```python
from build123d import *

# Parameters (mm, degrees)
SKETCH2_W                   = 42
SKETCH2_H                   = 42
MAIN_BOSS_DEPTH             = 33.75
SKETCH4_W                   = 8.7
SKETCH4_H                   = 17
SIDE_EXTRUDE_DEPTH          = 10
SKETCH5_R                   = 16.5
BIG_CIRCLE_CUT_DEPTH        = 0.5
SKETCH6_R                   = 11
MEDIUM_CIRCLE_EXTRUDE_DEPTH = 2.5
SKETCH7_R                   = 3.5
SMALL_CIRCLE_CUT_DEPTH      = 5
SKETCH8_R                   = 2.25
CIRCULAR_TALL_EXTRUDE_DEPTH = 23
SIDE_EDGE_CUT_DEPTH         = 50.62008162
MIRROR2_DEPTH               = 33.75
SKETCH10_R                  = 1.5
F_4_HOLES_DEPTH             = 5
MIRROR4_COPY_1_SKETCH_R     = 1.5
MIRROR4_COPY_1_DEPTH        = 5
MIRROR6_COPY_1_SKETCH_R     = 1.5
MIRROR6_COPY_1_DEPTH        = 5
MIRROR6_COPY_2_SKETCH_R     = 1.5
MIRROR6_COPY_2_DEPTH        = 5
MIRROR6_COPY_3_SKETCH_R     = 1.5
MIRROR6_COPY_3_DEPTH        = 5
SKETCH12_OUTSIDE_W          = 69.698
SKETCH12_OUTSIDE_H          = 60.998
CUT_AROUND_BODY_DEPTH       = 21


# Read off the part's stored shape, not the designer's step: Mirror2
with BuildPart() as part:
    # Sketch2 → Main Boss (new body)
    with BuildSketch(Plane(origin=(0, 0, 0), x_dir=(1, 0, 0), z_dir=(0, 1, 0))):
        Rectangle(SKETCH2_W, SKETCH2_H)
    extrude(amount=MAIN_BOSS_DEPTH)

    # Sketch4 → side extrude (add)
    with BuildSketch(Plane(origin=(0, 0, 0), x_dir=(1, 0, 0), z_dir=(0, 1, 0))):
        with Locations((25.35, 0)):
            Rectangle(SKETCH4_W, SKETCH4_H)
    extrude(amount=SIDE_EXTRUDE_DEPTH)

    # Sketch5 → Big circle cut (cut)
    with BuildSketch(Plane(origin=(0, 33.75, 0), x_dir=(1, 0, 0), z_dir=(0, 1, 0))):
        with Locations(Location((0, 0, 0), (0, 0, 270))):
            Circle(SKETCH5_R)
    extrude(amount=-BIG_CIRCLE_CUT_DEPTH, mode=Mode.SUBTRACT)

    # Sketch6 → medium circle extrude (add)
    with BuildSketch(Plane(origin=(0, 33.25, 0), x_dir=(1, 0, 0), z_dir=(0, 1, 0))):
        with Locations(Location((0, 0, 0), (0, 0, 270))):
            Circle(SKETCH6_R)
    extrude(amount=MEDIUM_CIRCLE_EXTRUDE_DEPTH)

    # Sketch7 → small circle cut (cut)
    with BuildSketch(Plane(origin=(0, 35.75, 0), x_dir=(1, 0, 0), z_dir=(0, 1, 0))):
        with Locations(Location((0, 0, 0), (0, 0, 270))):
            Circle(SKETCH7_R)
    extrude(amount=-SMALL_CIRCLE_CUT_DEPTH, mode=Mode.SUBTRACT)

    # Sketch8 → circular tall extrude (add)
    with BuildSketch(Plane(origin=(0, 30.75, 0), x_dir=(1, 0, 0), z_dir=(0, 1, 0))):
        with Locations(Location((0, 0, 0), (0, 0, 270))):
            Circle(SKETCH8_R)
    extrude(amount=CIRCULAR_TALL_EXTRUDE_DEPTH)

    # Sketch9 → side edge cut (cut, symmetric)
    with BuildSketch(Plane(origin=(0, 33.75, 0), x_dir=(1, 0, 0), z_dir=(0, 1, 0))):
        Polygon((79.674907888, 117.679754574), (-17.004846686, 21), (-21, 17.004846686), (-117.679754574, -79.674907888), (-311.039263723, 113.684601261), (-113.684601261, 311.039263723), align=None)
    side_edge_cut = extrude(amount=SIDE_EDGE_CUT_DEPTH, both=True, mode=Mode.SUBTRACT)

    # Mirror1: side edge cut across plane
    add(side_edge_cut.mirror(Plane.XY), mode=Mode.SUBTRACT)

    # Mirror2 outline → Mirror2 (cut)
    with BuildSketch(Plane(origin=(0, 0, 0), x_dir=(1, 0, 0), z_dir=(0, 1, 0))):
        Polygon((21, -21), (21, -17.004846686), (17.004846686, -21), align=None)
        Polygon((17.004846686, 21), (21, 17.004846686), (21, 21), align=None)
    extrude(amount=MIRROR2_DEPTH, mode=Mode.SUBTRACT)

    # Sketch10 → 4 holes (cut)
    with BuildSketch(Plane(origin=(0, 33.75, 0), x_dir=(1, 0, 0), z_dir=(0, 1, 0))):
        with Locations(Location((-15.5, 15.5, 0), (0, 0, 270))):
            Circle(SKETCH10_R)
    f_4_holes = extrude(amount=-F_4_HOLES_DEPTH, mode=Mode.SUBTRACT)

    # Mirror3: 4 holes across plane
    add(f_4_holes.mirror(Plane.XY), mode=Mode.SUBTRACT)

    # Mirror4: 4 holes across plane
    add(f_4_holes.mirror(Plane(origin=(0, 0, 0), x_dir=(0, 0, 1), z_dir=(1, 0, 0))), mode=Mode.SUBTRACT)

    # Mirror4 copy 1 sketch → Mirror4 copy 1 (cut)
    with BuildSketch(Plane(origin=(0, 33.75, 0), x_dir=(-1, 0, 0), z_dir=(0, 1, 0))):
        with Locations(Location((-15.5, 15.5, 0), (0, 0, 270))):
            Circle(MIRROR4_COPY_1_SKETCH_R)
    extrude(amount=-MIRROR4_COPY_1_DEPTH, mode=Mode.SUBTRACT)

    # Mirror6: 4 holes across plane
    add(f_4_holes.mirror(Plane.ZX.offset(16.875)), mode=Mode.SUBTRACT)

    # Mirror6 copy 1 sketch → Mirror6 copy 1 (cut)
    with BuildSketch(Plane.XZ):
        with Locations(Location((-15.5, 15.5, 0), (0, 0, 270))):
            Circle(MIRROR6_COPY_1_SKETCH_R)
    extrude(amount=-MIRROR6_COPY_1_DEPTH, mode=Mode.SUBTRACT)

    # Mirror6 copy 2 sketch → Mirror6 copy 2 (cut)
    with BuildSketch(Plane(origin=(0, 0, 0), x_dir=(-1, 0, 0), z_dir=(0, -1, 0))):
        with Locations(Location((-15.5, 15.5, 0), (0, 0, 270))):
            Circle(MIRROR6_COPY_2_SKETCH_R)
    extrude(amount=-MIRROR6_COPY_2_DEPTH, mode=Mode.SUBTRACT)

    # Mirror6 copy 3 sketch → Mirror6 copy 3 (cut)
    with BuildSketch(Plane(origin=(0, 0, 0), x_dir=(-1, 0, 0), z_dir=(0, -1, 0))):
        with Locations((-15.5, -15.5)):
            Circle(MIRROR6_COPY_3_SKETCH_R)
    extrude(amount=-MIRROR6_COPY_3_DEPTH, mode=Mode.SUBTRACT)

    # Sketch12 outside → cut around body (cut)
    with BuildSketch(Plane(origin=(0, 7, 0), x_dir=(1, 0, 0), z_dir=(0, 1, 0))):
        with Locations((4.35, 0)):
            Rectangle(SKETCH12_OUTSIDE_W, SKETCH12_OUTSIDE_H)
        with BuildLine():
            Line((-15.5, -19.5), (15.5, -19.5))
            ThreePointArc((15.5, -19.5), (18.328427125, -18.328427125), (19.5, -15.5))
            Line((19.5, -15.5), (19.5, 15.5))
            ThreePointArc((19.5, 15.5), (18.328427125, 18.328427125), (15.5, 19.5))
            Line((15.5, 19.5), (-15.5, 19.5))
            ThreePointArc((-15.5, 19.5), (-18.328427125, 18.328427125), (-19.5, 15.5))
            Line((-19.5, 15.5), (-19.5, -15.5))
            ThreePointArc((-19.5, -15.5), (-18.328427125, -18.328427125), (-15.5, -19.5))
        make_face(mode=Mode.SUBTRACT)
    extrude(amount=CUT_AROUND_BODY_DEPTH, mode=Mode.SUBTRACT)


solid = part.part
```
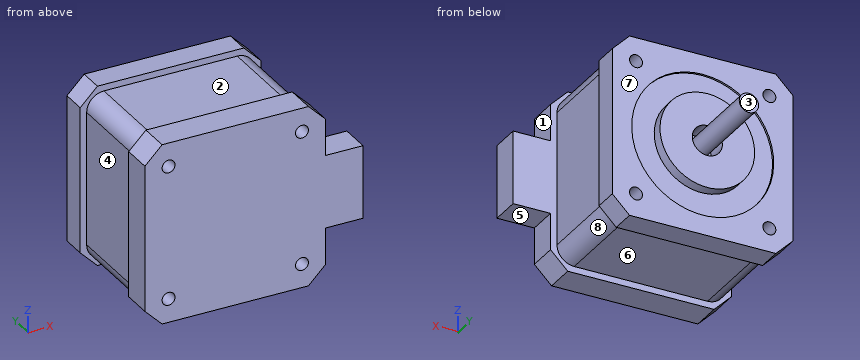
Read the model definition and answer for the solid it produces. Units are mm, in the model's axes. Face numbers are marked on the shaded views. A direction names the side the tool comes from. Give positions to 0.01 mm unless a question says otherwise; leave off trailing zeros. Write each loop counter-clockwise with the first axis right and the second up, starting at its lowest first coordinate (ties: lowest second). Pieces come first, ordered by that corner, then holes. Notation, with made-up numbers: (-34, -39) -> (0, -39) arc R21 cw to (0, -5) -> close; hole circle Ø2 at (60, 77). An arc over 180 degrees is marked (long way). Answer as a JSON object with one key per item and string values.
1) Section A-A on z = 0 is taken. Write down the section's boundary in (x, y).
Findings below:
{"outline": "(-21, 0) -> (29.7, 0) -> (29.7, 7) -> (19.5, 7) -> (19.5, 28) -> (21, 28) -> (21, 33.75) -> (16.5, 33.75) -> (16.5, 33.25) -> (11, 33.25) -> (11, 35.75) -> (3.5, 35.75) -> (3.5, 30.75) -> (2.25, 30.75) -> (2.25, 53.75) -> (-2.25, 53.75) -> (-2.25, 30.75) -> (-3.5, 30.75) -> (-3.5, 35.75) -> (-11, 35.75) -> (-11, 33.25) -> (-16.5, 33.25) -> (-16.5, 33.75) -> (-21, 33.75) -> (-21, 28) -> (-19.5, 28) -> (-19.5, 7) -> (-21, 7) -> close"}
2) For a pull along Y with two mould halves and no side action, classify the marked faces 1, 2, 3 and 4 as pulls with the +Y half, pulls with the -Y half, needs draft (parallel to the pull), parting line crosses it, or undercut.
Findings below:
{"face 1": "needs draft", "face 2": "undercut", "face 3": "pulls with the +Y half", "face 4": "undercut"}
3) Section D-D on z = -7 is taken. Write down the section's boundary in (x, y), then the cut area to 3 significant figures.
Findings below:
{"outline": "(-21, 0) -> (29.7, 0) -> (29.7, 7) -> (19.5, 7) -> (19.5, 28) -> (21, 28) -> (21, 33.75) -> (14.94, 33.75) -> (14.94, 33.25) -> (8.49, 33.25) -> (8.49, 35.75) -> (-8.49, 35.75) -> (-8.49, 33.25) -> (-14.94, 33.25) -> (-14.94, 33.75) -> (-21, 33.75) -> (-21, 28) -> (-19.5, 28) -> (-19.5, 7) -> (-21, 7) -> close", "area": "1,440 mm^2"}
4) Flat-ended cylindrical pins translate along their axes: pin 1 Ø3.5 at (x, z) = (-15.5, -15.5) entering from -Y; pin 2 Ø5 at (x, y) = (-2.5, 39) entering from -Z; pin 3 Ø0.9 at (x, z) = (-15, -15) entering from -Y; pin 4 Ø3 at (y, z) = (32, -1.5) entering from +X. Find the tip coordinate at first contact, or state that the pin passes through.
Findings below:
{"pin 1": "stops at y = 0", "pin 2": "stops at z = -2.25", "pin 3": "stops at y = 5", "pin 4": "stops at x = 21"}
5) Straight lines are drawn through the part: probe 1 along X at (y, z) = (3.7, -15.5); probe 2 along X at (y, z) = (32.5, 0). For each, find the intervals that lie inside material, in ascending order. Write a range as from..to.
Findings below:
{"probe 1": "x = -21..-17, -14..14, 17..21", "probe 2": "x = -21..-3.5, -2.25..2.25, 3.5..21"}
6) Section B-B on x = 0 is taken. Write down the section's boundary in (y, z).
Findings below:
{"outline": "(0, -21) -> (7, -21) -> (7, -19.5) -> (28, -19.5) -> (28, -21) -> (33.75, -21) -> (33.75, -16.5) -> (33.25, -16.5) -> (33.25, -11) -> (35.75, -11) -> (35.75, -3.5) -> (30.75, -3.5) -> (30.75, -2.25) -> (53.75, -2.25) -> (53.75, 2.25) -> (30.75, 2.25) -> (30.75, 3.5) -> (35.75, 3.5) -> (35.75, 11) -> (33.25, 11) -> (33.25, 16.5) -> (33.75, 16.5) -> (33.75, 21) -> (28, 21) -> (28, 19.5) -> (7, 19.5) -> (7, 21) -> (0, 21) -> close"}
7) Section C-C on y = 13.5 is taken. Write down the section's boundary in (x, z).
Findings below:
{"outline": "(-19.5, -15.5) arc R4 ccw to (-15.5, -19.5) -> (15.5, -19.5) arc R4 ccw to (19.5, -15.5) -> (19.5, 15.5) arc R4 ccw to (15.5, 19.5) -> (-15.5, 19.5) arc R4 ccw to (-19.5, 15.5) -> close"}
8) A tool of negligible diameter and unlimited length cuts with its end or side. For the marked faces 5, 6, 7 and 8, from which of +Z, -Z, +X, -X, +Y, -Y can it reach the whole face along a straight path? Write none if from no direction.
Findings below:
{"face 5": "-Z, +X, +Y, -Y", "face 6": "-Z, +X, -X", "face 7": "+Y", "face 8": "-Z, +X"}
